```python
from build123d import *

# Parameters (mm, degrees)
SKETCH1_R           = 12.5
SKETCH1_W           = 10
SKETCH1_H           = 70.75
SKETCH1_W_2         = 30
SKETCH1_H_2         = 6.5
BOSS_EXTRUDE1_DEPTH = 6.5
CUT_EXTRUDE1_REACH  = 146.217
SKETCH2_R           = 3.5
SKETCH2_3_R         = 8
SKETCH2_3_R_2       = 3.5
CUT_EXTRUDE2_DEPTH  = 4
CUT_EXTRUDE4_REACH  = 146.217
SKETCH3_R           = 2
CUT_EXTRUDE6_REACH  = 146.217
SKETCH5_R           = 2


with BuildPart() as part:
    # Sketch1 → Boss-Extrude1 (new body)
    with BuildSketch(Plane.XY):
        with Locations((0, 100)):
            Circle(SKETCH1_R)
        with BuildLine():
            Line((-48.897023427, 0), (48.897023427, 0))
            Line((48.897023427, 0), (12.5, 100))
            ThreePointArc((12.5, 100), (10.716279715, 93.564834962), (5.87418415, 88.966235431))
            Line((5.87418415, 88.966235431), (34.615543359, 10))
            Line((34.615543359, 10), (-34.615543359, 10))
            Line((-34.615543359, 10), (-5.87418415, 88.966235431))
            ThreePointArc((-5.87418415, 88.966235431), (-10.716279715, 93.564834962), (-12.5, 100))
            Line((-12.5, 100), (-48.897023427, 0))
        make_face()
        with BuildLine():
            Line((-5, 10), (5, 10))
            Line((5, 10), (5, 88.543560763))
            ThreePointArc((5, 88.543560763), (0, 87.5), (-5, 88.543560763))
            Line((-5, 88.543560763), (-5, 10))
        make_face()
        with Locations((85, 35.375)):
            Rectangle(SKETCH1_W, SKETCH1_H)
        with Locations((65, 15.5)):
            Rectangle(SKETCH1_W_2, SKETCH1_H_2)
        with Locations((65, 64)):
            Rectangle(SKETCH1_W_2, SKETCH1_H_2)
        with Locations((45, 35.375)):
            Rectangle(SKETCH1_W, SKETCH1_H)
    extrude(amount=BOSS_EXTRUDE1_DEPTH)

    # Sketch2 → Cut-Extrude1 (cut, up to next)
    with BuildSketch(Plane.XY.offset(6.5), mode=Mode.PRIVATE) as cut_extrude1_sk1:
        with Locations((0, 100)):
            Circle(SKETCH2_R)
    cut_extrude1_tool1 = extrude(cut_extrude1_sk1.sketch, amount=-CUT_EXTRUDE1_REACH, mode=Mode.PRIVATE) & part.part
    add(cut_extrude1_tool1.solids().sort_by_distance((0, 100, 6.5))[0], mode=Mode.SUBTRACT)

    # Sketch2_3 → Cut-Extrude2 (cut)
    with BuildSketch(Plane.XY.offset(6.5)):
        with Locations((0, 100)):
            Circle(SKETCH2_3_R)
        with Locations((0, 100)):
            Circle(SKETCH2_3_R_2, mode=Mode.SUBTRACT)
    extrude(amount=-CUT_EXTRUDE2_DEPTH, mode=Mode.SUBTRACT)

    # Sketch3 → Cut-Extrude4 (cut, up to next)
    with BuildSketch(Plane.XY.offset(6.5), mode=Mode.PRIVATE) as cut_extrude4_sk1:
        with Locations((-40.397023427, 5)):
            Circle(SKETCH3_R)
    cut_extrude4_tool1 = extrude(cut_extrude4_sk1.sketch, amount=-CUT_EXTRUDE4_REACH, mode=Mode.PRIVATE) & part.part
    # Sketch3 → Cut-Extrude4 (cut, up to next)
    with BuildSketch(Plane.XY.offset(6.5), mode=Mode.PRIVATE) as cut_extrude4_sk2:
        with Locations((0, 5)):
            Circle(SKETCH3_R)
    cut_extrude4_tool2 = extrude(cut_extrude4_sk2.sketch, amount=-CUT_EXTRUDE4_REACH, mode=Mode.PRIVATE) & part.part
    # Sketch3 → Cut-Extrude4 (cut, up to next)
    with BuildSketch(Plane.XY.offset(6.5), mode=Mode.PRIVATE) as cut_extrude4_sk3:
        with Locations((40.397023427, 5)):
            Circle(SKETCH3_R)
    cut_extrude4_tool3 = extrude(cut_extrude4_sk3.sketch, amount=-CUT_EXTRUDE4_REACH, mode=Mode.PRIVATE) & part.part
    # Sketch3 → Cut-Extrude4 (cut, up to next)
    with BuildSketch(Plane.XY.offset(6.5), mode=Mode.PRIVATE) as cut_extrude4_sk4:
        with Locations((0, 25)):
            Circle(SKETCH3_R)
    cut_extrude4_tool4 = extrude(cut_extrude4_sk4.sketch, amount=-CUT_EXTRUDE4_REACH, mode=Mode.PRIVATE) & part.part
    # Sketch3 → Cut-Extrude4 (cut, up to next)
    with BuildSketch(Plane.XY.offset(6.5), mode=Mode.PRIVATE) as cut_extrude4_sk5:
        with Locations((85, 5)):
            Circle(SKETCH3_R)
    cut_extrude4_tool5 = extrude(cut_extrude4_sk5.sketch, amount=-CUT_EXTRUDE4_REACH, mode=Mode.PRIVATE) & part.part
    add(cut_extrude4_tool1.solids().sort_by_distance((-40.397023, 5, 6.5))[0], mode=Mode.SUBTRACT)
    add(cut_extrude4_tool2.solids().sort_by_distance((0, 5, 6.5))[0], mode=Mode.SUBTRACT)
    add(cut_extrude4_tool3.solids().sort_by_distance((40.397023, 5, 6.5))[0], mode=Mode.SUBTRACT)
    add(cut_extrude4_tool4.solids().sort_by_distance((0, 25, 6.5))[0], mode=Mode.SUBTRACT)
    add(cut_extrude4_tool5.solids().sort_by_distance((85, 5, 6.5))[0], mode=Mode.SUBTRACT)

    # Sketch5 → Cut-Extrude6 (cut, up to next)
    with BuildSketch(Plane.XY.offset(6.5), mode=Mode.PRIVATE) as cut_extrude6_sk1:
        with Locations((60, 64)):
            Circle(SKETCH5_R)
    cut_extrude6_tool1 = extrude(cut_extrude6_sk1.sketch, amount=-CUT_EXTRUDE6_REACH, mode=Mode.PRIVATE) & part.part
    # Sketch5 → Cut-Extrude6 (cut, up to next)
    with BuildSketch(Plane.XY.offset(6.5), mode=Mode.PRIVATE) as cut_extrude6_sk2:
        with Locations((70, 64)):
            Circle(SKETCH5_R)
    cut_extrude6_tool2 = extrude(cut_extrude6_sk2.sketch, amount=-CUT_EXTRUDE6_REACH, mode=Mode.PRIVATE) & part.part
    # Sketch5 → Cut-Extrude6 (cut, up to next)
    with BuildSketch(Plane.XY.offset(6.5), mode=Mode.PRIVATE) as cut_extrude6_sk3:
        with Locations((70, 15.5)):
            Circle(SKETCH5_R)
    cut_extrude6_tool3 = extrude(cut_extrude6_sk3.sketch, amount=-CUT_EXTRUDE6_REACH, mode=Mode.PRIVATE) & part.part
    # Sketch5 → Cut-Extrude6 (cut, up to next)
    with BuildSketch(Plane.XY.offset(6.5), mode=Mode.PRIVATE) as cut_extrude6_sk4:
        with Locations((60, 15.5)):
            Circle(SKETCH5_R)
    cut_extrude6_tool4 = extrude(cut_extrude6_sk4.sketch, amount=-CUT_EXTRUDE6_REACH, mode=Mode.PRIVATE) & part.part
    add(cut_extrude6_tool1.solids().sort_by_distance((60, 64, 6.5))[0], mode=Mode.SUBTRACT)
    add(cut_extrude6_tool2.solids().sort_by_distance((70, 64, 6.5))[0], mode=Mode.SUBTRACT)
    add(cut_extrude6_tool3.solids().sort_by_distance((70, 15.5, 6.5))[0], mode=Mode.SUBTRACT)
    add(cut_extrude6_tool4.solids().sort_by_distance((60, 15.5, 6.5))[0], mode=Mode.SUBTRACT)


solid = part.part
```
Geometry: final body of the model. Coordinates: model frame, mm. A direction names the side the tool comes from. Give positions to 0.01 mm unless a question says otherwise; leave off trailing zeros. Write each loop counter-clockwise with the first axis right and the second up, starting at its lowest first coordinate (ties: lowest second). Pieces come first, ordered by that corner, then holes.
1. Section query B-B, the plane x = 85. Return loops of the section in (y, z).
2. Line query: probe 1 along Y at (x, z) = (0, 4.25); probe 2 along Y at (x, z) = (60, 3); probe 3 along Y at (x, z) = (74, 1.5). Output: solid intervals per line, ascending.
3. Reachability of faces 4 (the flat face through (25, 44, 6.5)), 5 (the flat face through (-5, 50, 3)), 6 (the flat face through (85, 70.75, 3)), 7 (the flat face through (80, 69, 3)), 8 (the flat face through (90, 35, 3)) from +Z, -Z, +X, -X, +Y, -Y: full face, straight path, thin tool, end or side. Return the list, or none.
4. Pin query (flat end, axial travel): P1, Ø2, axis at x = 63, z = 3, coming from the +Y side; P2, Ø3, axis at y = 53.5, z = 4.5, coming from the -X side; P3, Ø2, axis at y = 41.5, z = 4.5, coming from the -X side. Return the tip coordinate at first contact, or that it passes through.
5. Section query C-C, the plane y = 5. Return loops of the section in (x, z).
6. Draft query along Y for faces 1 (the flat face through (80, 6, 3)), 2 (the cylindrical face through (0.275, 112.497, 3.204)), 3 (the flat face through (20, 10, 3)). Return one class per face: released by +Y, released by -Y, zero draft, split by the parting line, or undercut.
7. Section query A-A, the plane x = 0. Return loops of the section in (y, z).
8. Section query D-D, the plane y = 46.5. Return loops of the section in (x, z), then the cut area to 3 significant figures.
Computed:
1. outline: (0, 0) - (3, 0) - (3, 6.5) - (0, 6.5) - close; (7, 0) - (70.75, 0) - (70.75, 6.5) - (7, 6.5) - close
2. probe 1: y = 0 to 3, 7 to 23, 27 to 92, 108 to 112.5
2. probe 2: y = 12.25 to 13.5, 17.5 to 18.75, 60.75 to 62, 66 to 67.25
2. probe 3: y = 12.25 to 18.75, 60.75 to 67.25
3. face 4: +Z, +X, -X, +Y, -Y
3. face 5: +Z, -Z
3. face 6: +Z, -Z, +X, +Y
3. face 7: +Z, -Z, +Y
3. face 8: +Z, -Z, +X, +Y, -Y
4. P1: stops at y = 67.25
4. P2: stops at x = -29.97
4. P3: stops at x = -34.16
5. outline: (-47.08, 0) - (-42.4, 0) - (-42.4, 6.5) - (-47.08, 6.5) - close; (-38.4, 0) - (-2, 0) - (-2, 6.5) - (-38.4, 6.5) - close; (2, 0) - (38.4, 0) - (38.4, 6.5) - (2, 6.5) - close; (42.4, 0) - (50, 0) - (50, 6.5) - (42.4, 6.5) - close; (80, 0) - (83, 0) - (83, 6.5) - (80, 6.5) - close; (87, 0) - (90, 0) - (90, 6.5) - (87, 6.5) - close
6. face 1: zero draft
6. face 2: released by +Y
6. face 3: undercut
7. outline: (0, 0) - (3, 0) - (3, 6.5) - (0, 6.5) - close; (7, 0) - (23, 0) - (23, 6.5) - (7, 6.5) - close; (27, 0) - (96.5, 0) - (96.5, 2.5) - (92, 2.5) - (92, 6.5) - (27, 6.5) - close; (103.5, 0) - (112.5, 0) - (112.5, 6.5) - (108, 6.5) - (108, 2.5) - (103.5, 2.5) - close
8. outline: (-31.97, 0) - (-21.33, 0) - (-21.33, 6.5) - (-31.97, 6.5) - close; (-5, 0) - (5, 0) - (5, 6.5) - (-5, 6.5) - close; (21.33, 0) - (31.97, 0) - (31.97, 6.5) - (21.33, 6.5) - close; (40, 0) - (50, 0) - (50, 6.5) - (40, 6.5) - close; (80, 0) - (90, 0) - (90, 6.5) - (80, 6.5) - close
8. area: 333 mm2
